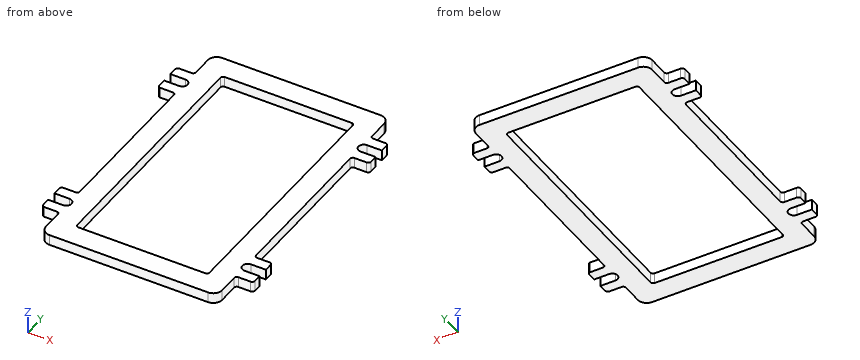
Autodesk Fusion 360 part; units mm, degrees
sketch "Sketch1" plane through (0, 0, 0) normal (0, 0, 1) x (1, 0, 0)
  line L0 (0, 0) -> (-90, 0)
  line L1 (0, 25) -> (-72, 25)
  line L2 (-75, 28) -> (-75, 165)
  arc A0 (-75, 28) -> (-72, 25) centre (-72, 28) ccw
  arc A1 (-100, 10) -> (-90, 0) centre (-90, 10) ccw
  line L3 (-103, 72) -> (-117, 72)
  line L4 (-120, 69) -> (-120, 39)
  line L5 (-117, 36) -> (-103, 36)
  line L6 (-120, 54) -> (-100, 54) construction
  line L7 (-103, 60) -> (-120, 60)
  line L8 (-120, 60) -> (-120, 48)
  line L9 (-120, 48) -> (-103, 48)
  arc A2 (-103, 48) -> (-103, 60) centre (-103, 54) ccw
  line L10 (-100, 10) -> (-100, 33)
  line L11 (-100, 75) -> (-100, 165)
  arc A3 (-117, 72) -> (-120, 69) centre (-117, 69) ccw
  arc A4 (-120, 39) -> (-117, 36) centre (-117, 39) ccw
  arc A5 (-103, 72) -> (-100, 75) centre (-103, 75) ccw
  arc A6 (-100, 33) -> (-103, 36) centre (-103, 33) ccw
  line L12 (0, 180) -> (0, -75.868) construction
  line L13 (75, 28) -> (75, 165)
  line L14 (103, 72) -> (117, 72)
  line L15 (0, 0) -> (90, 0)
  line L16 (103, 60) -> (120, 60)
  line L17 (120, 60) -> (120, 48)
  line L18 (100, 75) -> (100, 165)
  arc A7 (117, 36) -> (120, 39) centre (117, 39) ccw
  arc A8 (90, 0) -> (100, 10) centre (90, 10) ccw
  line L19 (100, 10) -> (100, 33)
  line L20 (120, 69) -> (120, 39)
  arc A9 (103, 60) -> (103, 48) centre (103, 54) ccw
  arc A10 (120, 69) -> (117, 72) centre (117, 69) ccw
  arc A11 (72, 25) -> (75, 28) centre (72, 28) ccw
  arc A12 (103, 36) -> (100, 33) centre (103, 33) ccw
  line L21 (120, 48) -> (103, 48)
  line L22 (0, 25) -> (72, 25)
  arc A13 (100, 75) -> (103, 72) centre (103, 75) ccw
  line L23 (120, 54) -> (100, 54) construction
  line L24 (117, 36) -> (103, 36)
  line L25 (100, 165) -> (-100, 165) construction
  line L26 (0, 150) -> (0, 405.868) construction
  line L27 (75, 302) -> (75, 165)
  line L28 (103, 258) -> (117, 258)
  line L29 (0, 305) -> (-72, 305)
  line L30 (-103, 270) -> (-120, 270)
  line L31 (120, 276) -> (100, 276) construction
  line L32 (-75, 302) -> (-75, 165)
  line L33 (0, 330) -> (90, 330)
  arc A14 (-103, 270) -> (-103, 282) centre (-103, 276) ccw
  line L34 (-103, 258) -> (-117, 258)
  arc A15 (-103, 294) -> (-100, 297) centre (-103, 297) ccw
  arc A16 (75, 302) -> (72, 305) centre (72, 302) ccw
  line L35 (-100, 320) -> (-100, 297)
  line L36 (-117, 294) -> (-103, 294)
  line L37 (-120, 261) -> (-120, 291)
  arc A17 (100, 320) -> (90, 330) centre (90, 320) ccw
  arc A18 (-72, 305) -> (-75, 302) centre (-72, 302) ccw
  line L38 (117, 294) -> (103, 294)
  arc A19 (117, 258) -> (120, 261) centre (117, 261) ccw
  arc A20 (-120, 261) -> (-117, 258) centre (-117, 261) ccw
  line L39 (120, 270) -> (120, 282)
  arc A21 (103, 282) -> (103, 270) centre (103, 276) ccw
  arc A22 (-90, 330) -> (-100, 320) centre (-90, 320) ccw
  arc A23 (-100, 255) -> (-103, 258) centre (-103, 255) ccw
  line L40 (-120, 270) -> (-120, 282)
  line L41 (120, 282) -> (103, 282)
  arc A24 (120, 291) -> (117, 294) centre (117, 291) ccw
  arc A25 (-117, 294) -> (-120, 291) centre (-117, 291) ccw
  line L42 (-120, 276) -> (-100, 276) construction
  arc A26 (100, 297) -> (103, 294) centre (103, 297) ccw
  line L43 (0, 330) -> (-90, 330)
  line L44 (-120, 282) -> (-103, 282)
  line L45 (100, 320) -> (100, 297)
  arc A27 (103, 258) -> (100, 255) centre (103, 255) ccw
  line L46 (103, 270) -> (120, 270)
  line L47 (120, 261) -> (120, 291)
  line L48 (-100, 255) -> (-100, 165)
  line L49 (100, 255) -> (100, 165)
  line L50 (0, 305) -> (72, 305)
  point P0 (-100, 0)
  point P1 (-75, 25)
  point P2 (-120, 72)
  point P3 (-120, 36)
  point P4 (120, 36)
  point P5 (120, 72)
  point P6 (100, 0)
  point P7 (75, 25)
  point P8 (-75, 305)
  point P9 (0, 330)
  point P10 (120, 258)
  point P11 (120, 294)
  point P12 (75, 305)
  point P13 (-100, 330)
  point P14 (-120, 294)
  point P15 (-120, 258)
  point P16 (100, 330)
  dimension "d16" = 100
  dimension "d17" = 165
  dimension "d18" = 25
  dimension "d19" = 25
  dimension "d20" = 140
  dimension "d21" = 3
  dimension "d22" = 10
  dimension "d23" = 12
  dimension "d24" = 3
  dimension "d25" = 36
  dimension "d28" = 3
  dimension "d29" = 3
  dimension "d30" = 3
  dimension "d31" = 54
  dimension "d32" = 36
extrude "Extrude1" add sketch "Sketch1" along normal blind 12 contours L0 A1 L3 L4 L5 L7 L9 A2 L10 L11 A3 A4 A5 A6 L14 L15 L16 L18 A7 A8 L19 L20 A9 A10 A12 L21 A13 L24 L28 L30 L33 A14 L34 A15 L35 L36 L37 A17 L38 A19 A20 A21 A22 A23 L41 A24 A25 A26 L43 L44 L45 A27 L46 L47 L48 L49
equation "width = 200 mm"
equation "length = 330 mm"
equation "outer_corner_radius = 10 mm"
equation "inner_corner_radius = 3 mm"
equation "edge_width = 25 mm"
equation "thickness = 12 mm"
equation "notch_diameter = 12 mm"
equation "notch_ear_extension = 20 mm"
equation "notch_ear_width = 12 mm"
equation "notch_inset = 3 mm"
equation "notch_to_edge_distance = 54 mm"
equation "d16 = width / 2"
equation "d17 = length / 2"
equation "d18 = edge_width"
equation "d19 = edge_width"
equation "d20 = ( length / 2 ) - ( edge_width )"
equation "d21 = inner_corner_radius"
equation "d22 = outer_corner_radius"
equation "d23 = notch_diameter"
equation "d24 = notch_inset"
equation "d25 = notch_diameter + ( notch_ear_width * 2 )"
equation "notch_ear_corner_radius = 3 mm"
equation "d28 = notch_ear_corner_radius"
equation "d29 = notch_ear_corner_radius"
equation "d30 = notch_ear_corner_radius"
equation "d31 = notch_to_edge_distance"
equation "d32 = notch_to_edge_distance - ( notch_diameter / 2 ) - notch_ear_width"
equation "d33 = thickness"
For this review, take the finished solid that the model builds, in its own axes (mm). Coordinates: 2 decimals unless noted, no trailing zeros. Write each loop counter-clockwise with the first axis right and the second up, starting at its lowest first coordinate (ties: lowest second). Pieces come first, ordered by that corner, then holes. Notation, with made-up numbers: (54, 70) -> (97, 70) arc R21 cw to (97, 94) -> close; hole circle Ø7 at (61, 81). An arc over 180 degrees is marked (long way). Write each question's results on one line, items separated by ' | '. Start each with the question number.
1) Insertion check: pin 1 (3.5 mm diameter, centred on x = -108, z = 6, fed in from -Y); pin 2 (3.5 mm diameter, centred on y = 23, z = 4, fed in from -X); pin 3 (3 mm diameter, centred on x = 91.5, z = 7.5, fed in from -Y); pin 4 (1 mm diameter, centred on y = 255.5, z = 7, fed in from -X). Each pin has a flat end and moves straight along its axis. Give the tip position at first contact, or say it passes through.
2) Wall thickness on L1, parallel to Y at x = 107, z = 11.25; L2, parallel to X at y = 175, z = 10.75; L3, parallel to X at y = 45, z = 3.25: over which ranges is each line inside the solid? List them lowest first. Write a range as [from, to].
3) Consider section B-B (x = -54). Write out the cut boundary in (y, z).
4) Consider section A-A (y = 100). Write out the cut boundary in (x, z).
Geometry says:
1) pin 1: y = 36 | pin 2: x = -100 | pin 3: y = 0 | pin 4: x = -100.17
2) L1: [36, 48], [60, 72], [258, 270], [282, 294] | L2: [-100, -75], [75, 100] | L3: [-120, -75], [75, 120]
3) outline: (0, 0) -> (25, 0) -> (25, 12) -> (0, 12) -> close; (305, 0) -> (330, 0) -> (330, 12) -> (305, 12) -> close
4) outline: (-100, 0) -> (-75, 0) -> (-75, 12) -> (-100, 12) -> close; (75, 0) -> (100, 0) -> (100, 12) -> (75, 12) -> close
